Design review of the part shown in the three views and the two pictorial views. Dimensions are in mm from the part's minimum x, y and z. A direction names the side the tool comes from. Round coordinates to 2 decimals unless told otherwise and drop trailing zeros. Loops run counter-clockwise (first coordinate to the right, second up) from the corner with the lowest first, then second, coordinate; pieces in that order, holes last. Notation, with made-up numbers: (-36.75, -25) -> (13.25, -25) arc R18 cw to (13.25, -18) -> close; hole circle Ø4 at (0.5, -29.75). An arc over 180 degrees is marked (long way). Write each question's results on one line, items separated by ' | '. Start each with the question number.
Item 1: Tool access review of the marked faces 1, 2 and 3: name each direction out of +Z, -Z, +X, -X, +Y, -Y from which nothing blocks a thin tool from reaching the whole face with its end or side.
Item 2: We need section C-C (z = 16.5). Give the boundary of the cut face in (x, y) (3 decimals), and give its area (4 significant figures).
Item 3: We need section A-A (y = 14). Give the boundary of the cut face in (x, z) (3 decimals).
Item 4: For L1, parallel to X at y = 14, z = 28.5 (3 decimals); L2, parallel to Z at x = 281.5, y = 18.5 (3 decimals); L3, parallel to X at y = 20.5, z = 24.5, list the stretches that pass through material, from the lowest coordinate up. Write a range as from..to.
Item 5: Clearance check with flat-ended pins moving along their axes: pin 1 Ø15 at (y, z) = (16, 33) entering from -X; pin 2 Ø5.5 at (x, z) = (285, 22.5) entering from -Y; pin 3 Ø11.5 at (x, y) = (9.5, 22.5) entering from +Z. State where each tip first meets the part, or that it passes through.
Item 6: We need section B-B (z = 33.5). Give the boundary of the cut face in (x, y).
Item 7: We need section D-D (x = 143). Give the boundary of the cut face in (y, z), and give its area (3 significant figures).
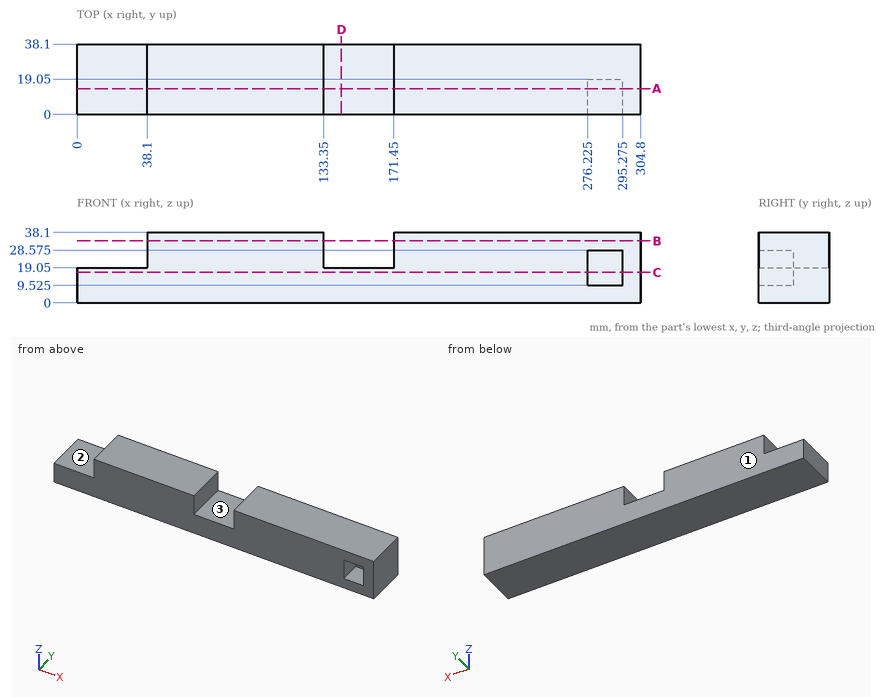
Here are the results:
1) face 1: +Z, -Z, +X, -X, +Y | face 2: +Z, -X, +Y, -Y | face 3: +Z, +Y, -Y
2) outline: (0, 0) -> (276.225, 0) -> (276.225, 19.05) -> (295.275, 19.05) -> (295.275, 0) -> (304.8, 0) -> (304.8, 38.1) -> (0, 38.1) -> close | area: 11,250 mm2
3) outline: (0, 0) -> (304.8, 0) -> (304.8, 38.1) -> (171.45, 38.1) -> (171.45, 19.05) -> (133.35, 19.05) -> (133.35, 38.1) -> (38.1, 38.1) -> (38.1, 19.05) -> (0, 19.05) -> close; hole (276.225, 9.525) -> (295.275, 9.525) -> (295.275, 28.575) -> (276.225, 28.575) -> close
4) L1: x = 38.1..133.35, 171.45..276.225, 295.275..304.8 | L2: z = 0..9.525, 28.575..38.1 | L3: x = 38.1..133.35, 171.45..304.8
5) pin 1: stops at x = 38.1 | pin 2: stops at y = 19.05 | pin 3: stops at z = 19.05
6) outline: (38.1, 0) -> (133.35, 0) -> (133.35, 38.1) -> (38.1, 38.1) -> close; (171.45, 0) -> (304.8, 0) -> (304.8, 38.1) -> (171.45, 38.1) -> close
7) outline: (0, 0) -> (38.1, 0) -> (38.1, 19.05) -> (0, 19.05) -> close | area: 726 mm2
